Build history of the part. All positions in model axes, mm. Face numbers are marked on the shaded views. A direction names the side the tool comes from. Coordinates: 2 decimals unless noted, no trailing zeros. Loops run counter-clockwise (first coordinate to the right, second up) from the corner with the lowest first, then second, coordinate; pieces in that order, holes last.
Item 1: Flat gauge pins, fed straight in: pin 1 (4 mm diameter, centred on y = -25.5, z = 3, fed in from -X); pin 2 (1.5 mm diameter, centred on x = 1.5, y = -61.5, fed in from +Z); pin 3 (2 mm diameter, centred on y = -33.5, z = -3.5, fed in from +X). Where does each tip first touch, or does it go through?
Item 2: Drill centre lines: line 1 along Y through (x, z) = (1.25, 6); line 2 along X through (y, z) = (-61, 0.25); line 3 along Z through (x, y) = (0, -72) (3 decimals). Where is each one in solid material? Low to high.
Item 3: Cut at C-C (y = -77). List the corners of the cut face in (x, z) (3 decimals), and give its area (3 significant figures).
Item 4: Cut at B-B (x = 0). List the corners of the cut face in (y, z) (3 decimals).
Item 5: 3-axis set-ups, long thin cutter, end or side, ignore diameter. For the marked faces 1 and 2: which of +Z, -Z, +X, -X, +Y, -Y reach the whole face in a straight line?
Item 6: Cut at D-D (y = -6). List the corners of the cut face in (x, z) (3 decimals), and give its area (3 significant figures).
Item 7: Cut at A-A (z = 0). List the corners of the cut face in (x, y) (3 decimals).
Autodesk Inventor part; units mm, degrees
ref_plane "YZ Plane" through (0, 0, 0) normal (1, 0, 0) x (0, 1, 0)
ref_plane "XZ Plane" through (0, 0, 0) normal (0, 1, 0) x (-1, 0, 0)
ref_plane "XY Plane" through (0, 0, 0) normal (0, 0, 1) x (1, 0, 0)
sketch "Sketch1" plane through (0, 0, 0) normal (0, 1, 0) x (-1, 0, 0)
  circle A0 centre (0, 0) radius 6.41
  dimension "d0" = 12.82
extrude "Extrusion1" add sketch "Sketch1" along normal blind 7.92
sketch "Sketch2" plane through (0, 7.92, 0) normal (0, 1, 0) x (1, 0, 0)
  circle A0 centre (0, 0) radius 3.905
  dimension "d3" = 7.81
extrude "Extrusion2" add sketch "Sketch2" against normal blind 98.1
sketch "Sketch3" plane through (0, -90.18, 0) normal (0, -1, 0) x (1, 0, 0)
  circle A0 centre (0, 0) radius 3.905
  circle A1 centre (0, 0) radius 3.905
  circle A2 centre (0, 0) radius 3.405
  dimension "d6" = 0.5
extrude "Extrusion3" cut sketch "Sketch3" against normal blind 30.75
properties part number "PlotterScrew"
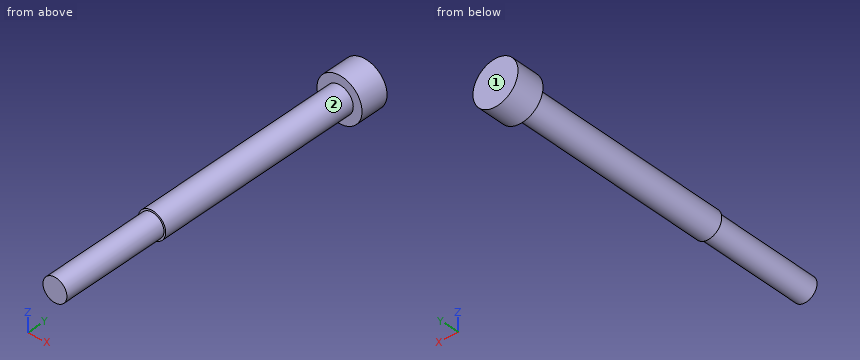
Filled sheet:
1. pin 1: stops at x = -3.77
1. pin 2: stops at z = 3.32
1. pin 3: stops at x = 3
2. line 1: y = 0 to 7.92
2. line 2: x = -3.4 to 3.4
2. line 3: z = -3.405 to 3.405
3. outline: circle Ø6.81 at (0, 0)
3. area: 36.4 mm2
4. outline: (-90.18, -3.405) - (-59.43, -3.405) - (-59.43, -3.905) - (0, -3.905) - (0, -6.41) - (7.92, -6.41) - (7.92, 6.41) - (0, 6.41) - (0, 3.905) - (-59.43, 3.905) - (-59.43, 3.405) - (-90.18, 3.405) - close
5. face 1: +Z, -Z, +X, -X, +Y
5. face 2: -Y
6. outline: circle Ø7.81 at (0, 0)
6. area: 47.9 mm2
7. outline: (-6.41, 0) - (-3.905, 0) - (-3.905, -59.43) - (-3.405, -59.43) - (-3.405, -90.18) - (3.405, -90.18) - (3.405, -59.43) - (3.905, -59.43) - (3.905, 0) - (6.41, 0) - (6.41, 7.92) - (-6.41, 7.92) - close
